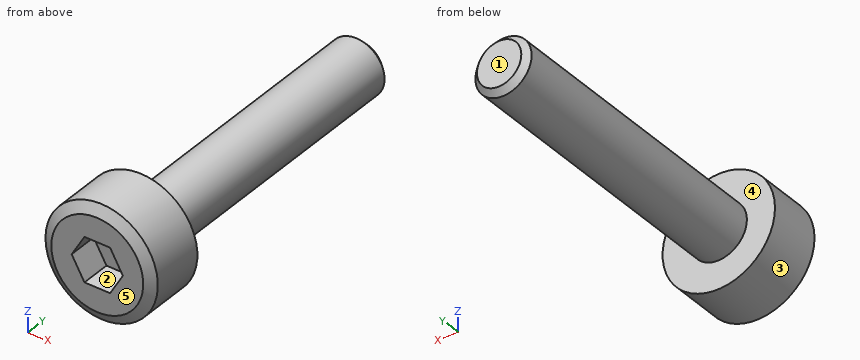
```python
from build123d import *

# Parameters (mm, degrees)
CUT_EXTRUDE1_DEPTH = 1


with BuildPart() as part:
    # Sketch1 → Base-Revolve (revolve)
    with BuildSketch(Plane.XY, mode=Mode.PRIVATE) as base_revolve_sk:
        Polygon((0.95, 0), (1.9, 0), (1.9, -1.8), (1.553589838, -2), (0, -2), (0, 10), (0.75, 10), (0.95, 9.8), align=None)
    revolve(base_revolve_sk.sketch.rotate(Axis((0, -2, 0), (0, -1, 0)), 180), axis=Axis((0, -2, 0), (0, -1, 0)))

    # Sketch2 → Cut-Extrude1 (cut)
    with BuildSketch(Plane.XZ.offset(2)):
        Polygon((-0.433012702, 0.75), (0.433012702, 0.75), (0.866025404, 0), (0.433012702, -0.75), (-0.433012702, -0.75), (-0.866025404, 0), align=None)
    extrude(amount=-CUT_EXTRUDE1_DEPTH, mode=Mode.SUBTRACT)


solid = part.part
```
The listing builds one solid part. Answer for the finished solid, in the listing's coordinates (mm). Face numbers are marked on the shaded views. A direction names the side the tool comes from. Round coordinates to 2 decimals unless told otherwise and drop trailing zeros. Loops run counter-clockwise (first coordinate to the right, second up) from the corner with the lowest first, then second, coordinate; pieces in that order, holes last.
1) A cutting plane is placed at B-B on y = -0.5. Determine the outline of the cut face in (x, z).
Outcome:
outline: circle Ø3.8 at (0, 0)
2) For a pull along Z with two mould halves and no side action, classify the marked faces 1, 2 and 3 as released by +Z, released by -Z, zero draft, split by the parting line, or undercut.
Outcome:
face 1: zero draft
face 2: undercut
face 3: split by the parting line
3) A cutting plane is placed at A-A on x = 0. Determine the outline of the cut face in (y, z).
Outcome:
outline: (-2, -1.55) - (-1.8, -1.9) - (0, -1.9) - (0, -0.95) - (9.8, -0.95) - (10, -0.75) - (10, 0.75) - (9.8, 0.95) - (0, 0.95) - (0, 1.9) - (-1.8, 1.9) - (-2, 1.55) - (-2, 0.75) - (-1, 0.75) - (-1, -0.75) - (-2, -0.75) - close
4) Consider line 1 (Z direction, x = 0, y = 1.75); line 2 (Y direction, x = 0.3, z = -0.5); line 3 (Y direction, x = -1.2, z = -0.75). Determine where each line is inside the solid, lowest interval first.
Outcome:
line 1: z = -0.95 to 0.95
line 2: y = -1 to 10
line 3: y = -2 to 0
5) Given P1, Ø1, axis at x = -1.5, y = 7, coming from the +Z side; P2, Ø1.5, axis at y = 0.5, z = -1, coming from the +X side, each flat-ended and moving along its own axis, determine where each tip first touches the part or whether it passes through.
Outcome:
P1: passes through
P2: stops at x = 1.85
6) A cutting plane is placed at C-C on y = 6.75. Determine the outline of the cut face in (x, z).
Outcome:
outline: circle Ø1.9 at (0, 0)
7) For the marked faces 4 and 5, determine the directions among +Z, -Z, +X, -X, +Y, -Y from which every point of the face is accessible in a straight line to the end or side of a thin tool.
Outcome:
face 4: +Y
face 5: +Z, -Z, +X, -X, -Y
